```python
from build123d import *

# Parameters (mm, degrees)
SKETCH1_W           = 22
SKETCH1_H           = 40
SKETCH1_R           = 1.760631049
SKETCH1_R_2         = 1.555398854
BOSS_EXTRUDE1_DEPTH = 5
BOSS_EXTRUDE3_DEPTH = 40
FILLET1_R           = 2
SKETCH6_R           = 1.5
CUT_EXTRUDE1_DEPTH  = 7.086873748


with BuildPart() as part:
    # Sketch1 → Boss-Extrude1 (new body)
    with BuildSketch(Plane(origin=(0, 0, 0), x_dir=(1, 0, 0), z_dir=(0, 1, 0))):
        Rectangle(SKETCH1_W, SKETCH1_H)
        with Locations(Location((0, 15, 0), (0, 0, 270))):
            Circle(SKETCH1_R, mode=Mode.SUBTRACT)
        with Locations(Location((0, -15, 0), (0, 0, 270))):
            Circle(SKETCH1_R_2, mode=Mode.SUBTRACT)
    extrude(amount=BOSS_EXTRUDE1_DEPTH)

    # Sketch4 → Boss-Extrude3 (add)
    with BuildSketch(Plane(origin=(0, 0, -20), x_dir=(-1, 0, 0), z_dir=(0, 0, -1))):
        Polygon((-11, 5), (-12, 5), (-12, 8.5), (-15, 8.5), (-15, 0), (-11, 0), align=None)
        Polygon((11, 0), (11, 5), (12, 5), (12, 8.5), (15, 8.5), (15, 0), align=None)
    extrude(amount=-BOSS_EXTRUDE3_DEPTH)

    # Fillet1
    fillet1_edges = [part.edges().sort_by_distance(p)[0] for p in [
        (15, 0, 0),
        (15, 8.5, 0),
        (-15, 0, 0),
        (-15, 8.5, 0),
    ]]
    fillet(fillet1_edges, radius=FILLET1_R)

    # Sketch2 → Loft1 section 0
    with BuildSketch(Plane.XZ):
        with BuildLine():
            Line((-11, 0.105117767), (11, 6))
            Line((11, 6), (11, -2))
            Line((11, -2), (-11, -7.894882233))
            Line((-11, -7.894882233), (-11, 0.105117767))
        make_face()
    # Sketch5 → Loft1 section 1
    with BuildSketch(Plane(origin=(0, -20, 0), x_dir=(-1, 0, 0), z_dir=(0, -1, 0))):
        with BuildLine():
            Line((-11, 3), (-11, 11))
            Line((-11, 11), (11, 16.894882233))
            Line((11, 16.894882233), (11, 8.894882233))
            Line((11, 8.894882233), (-11, 3))
        make_face()
    loft()

    # Sketch6 → Cut-Extrude1 (cut)
    with BuildSketch(Plane(origin=(1.040309356, 1.747119317, -3.882487372), x_dir=(0.9714204714250083, -0.09740631922929449, 0.21645848717621435), z_dir=(-0.2373652621939752, -0.3986366483069059, 0.8858592184598079))):
        with Locations(Location((5.252708211, -11.411685947, 0), (0, 0, 90))):
            Circle(SKETCH6_R)
        with Locations(Location((-7.39453945, -12.762593713, 0), (0, 0, 90))):
            Circle(SKETCH6_R)
    extrude(amount=CUT_EXTRUDE1_DEPTH, mode=Mode.SUBTRACT)


solid = part.part
```
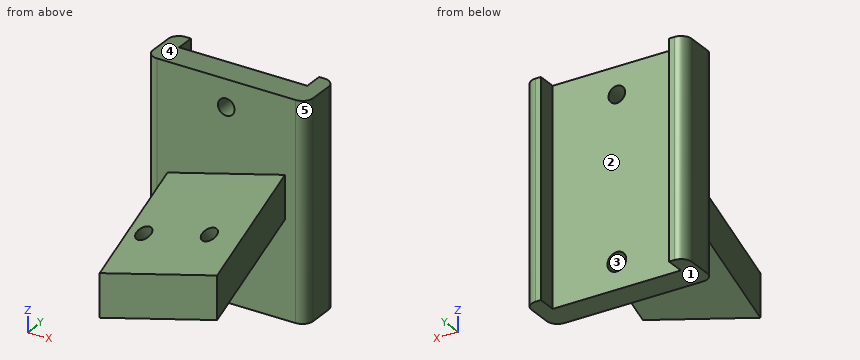
CAD build for the part. Positions are in the model's coordinates, mm. Face numbers are marked on the shaded views. A direction names the side the tool comes from. Give positions to 0.01 mm unless a question says otherwise; leave off trailing zeros. Order: outer loops, then holes, each group sorted by start corner. A loop starts at its lowest first (then second) coordinate and runs counter-clockwise, first axis right, second up.
(1) Drill centre lines: L1, parallel to X at y = 1.5, z = -14; L2, parallel to Y at x = -8.25, z = -10.5; L3, parallel to X at y = 3.7, z = -15. Where is each one in solid material? Low to high.
(2) Flat gauge pins, fed straight in: pin 1 (7 mm diameter, centred on x = 4.5, z = 5.5, fed in from +Y); pin 2 (12 mm diameter, centred on x = 9, y = -16, fed in from +Z); pin 3 (3 mm diameter, centred on x = 0, z = -15, fed in from +Y); pin 4 (12 mm diameter, centred on x = 2.5, y = 5.5, fed in from -Z). Where does each tip first touch, or does it go through?
(3) Mould opens along X. For the marked faces 3, 4 and 5 say: released by +X, released by -X, zero draft, split by the parting line, or undercut.
(4) Saw through at C-C, the plane x = 0. State how many separate pieces and enclosed holes the cut face has, then the cut area to 3 significant figures.
(5) Saw through at B-B, the plane y = 0.5. Give the cut face in (x, z).
(6) Saw through at A-A, the plane z = 15. Give the cut face in (x, y), then the cut area to 3 significant figures.
(7) Tool access for the marked faces 1 and 2: list every direction of +Z, -Z, +X, -X, +Y, -Y with a clear straight run to the whole face (end or side of a thin tool).
Results found:
1. L1: x = -14.94 to -1.45, 1.45 to 14.94
1. L2: y = -20 to -7.43, 0 to 5
1. L3: x = -15 to -1.76, 1.76 to 15
2. pin 1: stops at y = 5
2. pin 2: stops at z = 1.35
2. pin 3: stops at y = -18.89
2. pin 4: stops at z = -20
3. face 3: undercut
3. face 4: zero draft
3. face 5: released by +X
4. separate pieces: 3
4. enclosed holes: 0
4. area: 327 mm2
5. outline: (-14.32, -20) - (14.32, -20) - (14.32, 20) - (-14.32, 20) - close; hole circle Ø3.52 at (0, -15); hole circle Ø3.11 at (0, 15)
6. outline: (-15, 2) arc R2 ccw to (-13, 0) - (-1.56, 0) - (-1.56, 5) - (-12, 5) - (-12, 8.5) - (-13, 8.5) arc R2 ccw to (-15, 6.5) - close; (1.56, 0) - (13, 0) arc R2 ccw to (15, 2) - (15, 6.5) arc R2 ccw to (13, 8.5) - (12, 8.5) - (12, 5) - (1.56, 5) - close
6. area: 152 mm2
7. face 1: -Z, +X, -X, +Y, -Y
7. face 2: +Z, -Z, +Y
